Autodesk Inventor part; units mm, degrees
ref_plane "YZ Plane" through (0, 0, 0) normal (1, 0, 0) x (0, 1, 0)
ref_plane "XZ Plane" through (0, 0, 0) normal (0, 1, 0) x (-1, 0, 0)
ref_plane "XY Plane" through (0, 0, 0) normal (0, 0, 1) x (1, 0, 0)
sketch "Sketch1" plane through (0, 0, 0) normal (0, 1, 0) x (-1, 0, 0)
  line L0 (-1.9439, 0) -> (23.4561, 0)
  line L1 (23.4561, 0) -> (23.4561, 25.4)
  line L2 (23.4561, 25.4) -> (-1.9439, 25.4)
  line L3 (-1.9439, 25.4) -> (-1.9439, 0)
  line L4 (20.2811, 22.225) -> (1.2311, 22.225)
  line L5 (1.2311, 22.225) -> (1.2311, 3.175)
  line L6 (1.2311, 3.175) -> (20.2811, 3.175)
  line L7 (20.2811, 3.175) -> (20.2811, 22.225)
  point P0 (0, 0)
  dimension "d0" = 25.4
  dimension "d1" = 25.4
  dimension "d2" = 3.175
  dimension "d4" = 3.175
  dimension "d5" = 3.175
  dimension "d6" = 3.175
extrude "Extrusion1" add sketch "Sketch1" along normal blind 660.4
sketch "Sketch2" plane through (1.9439, 0, 25.4) normal (1, 0, 0) x (0, 0, -1)
  circle A0 centre (12.7, 12.7) radius 6.35
  line L0 (25.4, 0) -> (25.4, 660.4)
  line L1 (0, 0) -> (25.4, 0)
  circle A1 centre (12.7, 647.7) radius 6.35
  line L2 (0, 660.4) -> (25.4, 660.4)
  dimension "d9" = 12.7
  dimension "d10" = 12.7
  dimension "d11" = 12.7
  dimension "d12" = 12.7
  dimension "d13" = 12.7
  dimension "d14" = 12.7
extrude "Extrusion2" cut sketch "Sketch2" against normal blind 660.4
sketch "Sketch3" plane through (1.9439, 0, 25.4) normal (1, 0, 0) x (0, 0, -1)
  circle A0 centre (12.7, 647.7) radius 6.35
  circle A1 centre (12.7, 647.7) radius 6.35
  circle A2 centre (12.7, 12.7) radius 6.35
  circle A3 centre (12.7, 114.3) radius 6.35
  line L0 (0, 0) -> (25.4, 0)
  line L1 (25.4, 0) -> (25.4, 660.4)
  dimension "d17" = 12.7
  dimension "d18" = 12.7
  dimension "d19" = 12.7
  dimension "d20" = 12.7
  dimension "d21" = 101.6
  dimension "d22" = 12.7
extrude "Extrusion3" cut sketch "Sketch3" against normal blind 660.4 contours A3
sketch "Sketch4" plane through (-23.4561, 0, 25.4) normal (0, 0, 1) x (1, 0, 0)
  point P0 (23.4561, 0)
sketch "Sketch5" plane through (1.9439, 0, 25.4) normal (1, 0, 0) x (0, 0, -1)
  circle A0 centre (12.7, 215.9) radius 6.35
  circle A1 centre (12.7, 114.3) radius 6.35
  circle A2 centre (12.7, 114.3) radius 6.35
  line L0 (25.4, 0) -> (25.4, 660.4)
  dimension "d25" = 12.7
  dimension "d26" = 101.6
  dimension "d27" = 12.7
extrude "Extrusion4" cut sketch "Sketch5" against normal blind 660.4 contours A0
properties part number "26 inch 8th inch thick tube"
Could you check a few things on this model? Use its own coordinates, in mm. A direction names the side the tool comes from. Coordinates: 2 decimals unless noted, no trailing zeros. Write each loop counter-clockwise with the first axis right and the second up, starting at its lowest first coordinate (ties: lowest second). Pieces come first, ordered by that corner, then holes. Notation, with made-up numbers: (50.5, -15.75) - (108.5, -15.75) arc R28 ccw to (108.5, 7.25) - close; hole circle Ø10 at (61, -4). An arc over 180 degrees is marked (long way). Use a Markdown table: item, result.
Q1. Imagine slicing it at C-C (z = 12.7). Count the separate pieces of the cut face and the enclosed holes in it, and give its area (3 significant figures).
Geometry check:
| item | result |
|---|---|
| separate pieces | 10 |
| enclosed holes | 0 |
| area | 3,870 mm2 |
Q2. Please list where these lines run through material, in increasing order: L1, parallel to Y at x = 0.5, z = 12.7; L2, parallel to X at y = 314, z = 14.5; L3, parallel to Z at x = -3.5, y = 275 (3 decimals).
Geometry check:
| item | result |
|---|---|
| L1 | y = 0 to 6.35, 19.05 to 107.95, 120.65 to 209.55, 222.25 to 641.35, 654.05 to 660.4 |
| L2 | x = -23.46 to -20.28, -1.23 to 1.94 |
| L3 | z = 0 to 3.175, 22.225 to 25.4 |
Q3. Imagine slicing it at B-B (y = 114.3). List the corners of the cut face in (x, z) for me (3 decimals), and give its area (3 significant figures).
Geometry check:
| item | result |
|---|---|
| outline | (-23.456, 0) - (1.944, 0) - (1.944, 6.35) - (-1.231, 6.35) - (-1.231, 3.175) - (-20.281, 3.175) - (-20.281, 6.35) - (-23.456, 6.35) - close; (-23.456, 19.05) - (-20.281, 19.05) - (-20.281, 22.225) - (-1.231, 22.225) - (-1.231, 19.05) - (1.944, 19.05) - (1.944, 25.4) - (-23.456, 25.4) - close |
| area | 202 mm2 |
Q4. Thinking about a two-plate mould opening in Y: for faces 1 (the cylindrical face through (0.379, 18.054, 9.286)), 2 (the flat face through (1, 0, 13)), 3 (the flat face through (1.944, 326, 13)), which applies, +Y half, -Y half, draft (parallel to the pull), parting line (faces both ways), or undercut?
Geometry check:
| item | result |
|---|---|
| face 1 | undercut |
| face 2 | -Y half |
| face 3 | draft |
Q5. Which directions (+Z, -Z, +X, -X, +Y, -Y) give clear straight access to the entire face, cutting with the end or side of a thin tool? Please do faces 4 (the flat face through (-11, 326, 3.175)), 5 (the cylindrical face through (0.38, 108.1, 14.08)).
Geometry check:
| item | result |
|---|---|
| face 4 | +Y, -Y |
| face 5 | +X, -X |
Q6. Imagine slicing it at A-A (x = -15.5). List the corners of the cut face in (y, z) for me (3 decimals), and give its area (3 significant figures).
Geometry check:
| item | result |
|---|---|
| outline | (0, 0) - (660.4, 0) - (660.4, 3.175) - (0, 3.175) - close; (0, 22.225) - (660.4, 22.225) - (660.4, 25.4) - (0, 25.4) - close |
| area | 4,190 mm2 |
